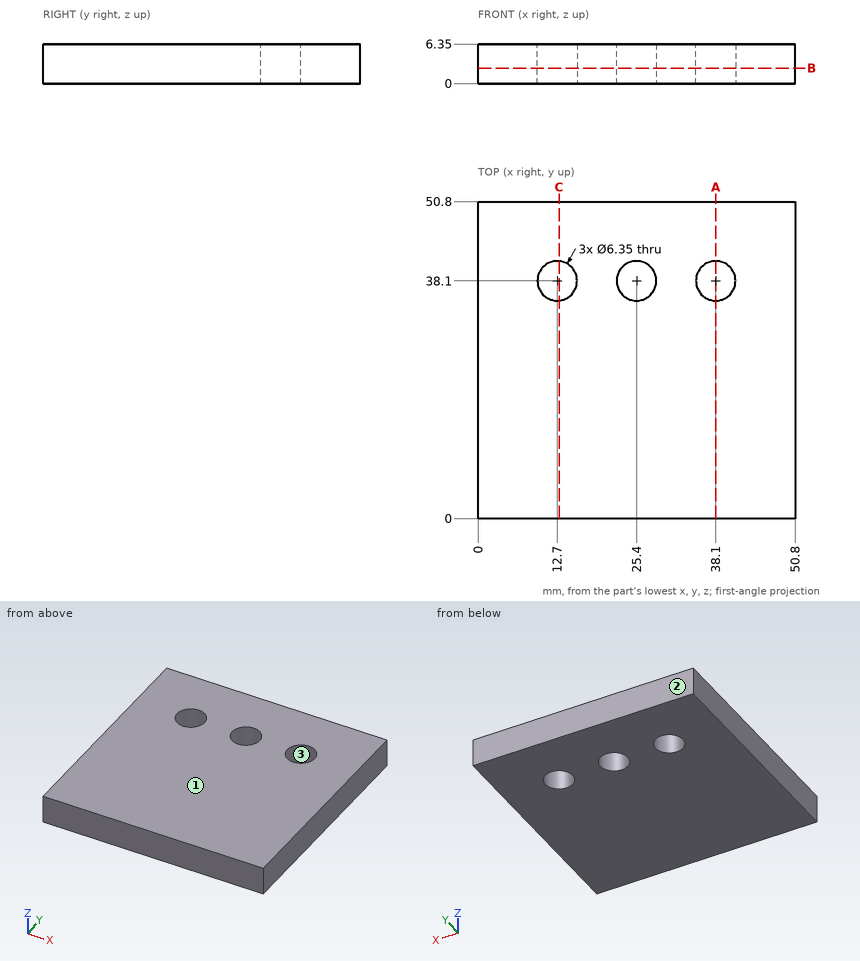
The drawing under review shows one solid part. Ordinate dimensions are in mm from its lowest x, y, z. Round coordinates to 2 decimals unless told otherwise and drop trailing zeros. Order: outer loops, then holes, each group sorted by start corner. A loop starts at its lowest first (then second) coordinate and runs counter-clockwise, first axis right, second up. Notation, with made-up numbers: (89.5, 0) -> (100.5, 0) arc R9 ccw to (100.5, 17) -> close; hole circle Ø5 at (63.5, -3.5). An arc over 180 degrees is marked (long way). Use a Markdown table: item, result.
Q1. We need section C-C on x = 13. Write out the cut boundary in (y, z), then the cut area to 3 significant figures.
Values:
| item | result |
|---|---|
| outline | (0, 0) -> (34.94, 0) -> (34.94, 6.35) -> (0, 6.35) -> close; (41.26, 0) -> (50.8, 0) -> (50.8, 6.35) -> (41.26, 6.35) -> close |
| area | 282 mm^2 |
Q2. Mouldability with a two-part tool opening along Y and no side actions: class the marked faces 1, 2 and 3 as +Y half, -Y half, draft (parallel to the pull), parting line (faces both ways), or undercut.
Values:
| item | result |
|---|---|
| face 1 | draft |
| face 2 | +Y half |
| face 3 | undercut |
Q3. We need section B-B on z = 2.5. Write out the cut boundary in (x, y) (3 decimals).
Values:
| item | result |
|---|---|
| outline | (0, 0) -> (50.8, 0) -> (50.8, 50.8) -> (0, 50.8) -> close; hole circle Ø6.35 at (12.7, 38.1); hole circle Ø6.35 at (25.4, 38.1); hole circle Ø6.35 at (38.1, 38.1) |
Q4. We need section A-A on x = 38.1. Write out the cut boundary in (y, z) (3 decimals).
Values:
| item | result |
|---|---|
| outline | (0, 0) -> (34.925, 0) -> (34.925, 6.35) -> (0, 6.35) -> close; (41.275, 0) -> (50.8, 0) -> (50.8, 6.35) -> (41.275, 6.35) -> close |
Q5. For line 1 (Y direction, x = 38.1, z = 2) (3 decimals); line 2 (X direction, y = 37.5, z = 5.25); line 3 (Y direction, x = 15, z = 2.75), list the stretches that pass through material, from the lowest coordinate up.
Values:
| item | result |
|---|---|
| line 1 | y = 0 to 34.925, 41.275 to 50.8 |
| line 2 | x = 0 to 9.58, 15.82 to 22.28, 28.52 to 34.98, 41.22 to 50.8 |
| line 3 | y = 0 to 35.91, 40.29 to 50.8 |
Q6. Clearance check with flat-ended pins moving along their axes: P1, Ø6, axis at x = 27, y = 29.5, coming from the -Z side; P2, Ø4, axis at x = 25.4, y = 38.1, coming from the +Z side. State where each tip first meets the part, or that it passes through.
Values:
| item | result |
|---|---|
| P1 | stops at z = 0 |
| P2 | passes through |
